Model file for the job. Use its own axes, mm. Face numbers are marked on the shaded views. A direction names the side the tool comes from. Round coordinates to 2 decimals unless told otherwise and drop trailing zeros. Loops run counter-clockwise (first coordinate to the right, second up) from the corner with the lowest first, then second, coordinate; pieces in that order, holes last. Notation, with made-up numbers: (-23.75, -28.75) -> (26.25, -28.75) arc R34 cw to (26.25, 3.25) -> close; hole circle Ø9 at (20, 25). An arc over 180 degrees is marked (long way). Use a Markdown table: item, result. Add a question column.
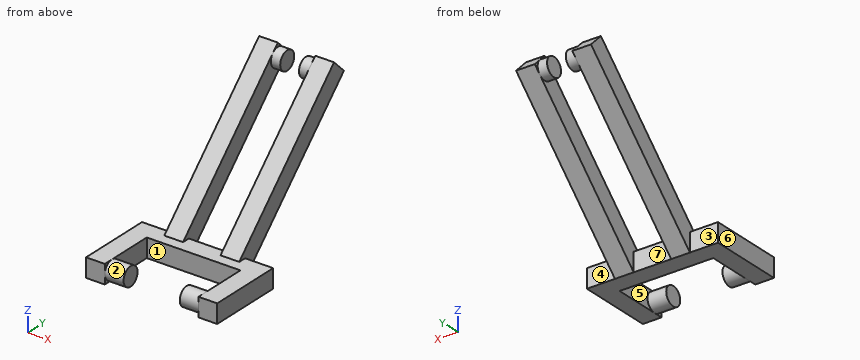
```python
from build123d import *

# Parameters (mm, degrees)
F1_DEPTH = 10
F2_R     = 5
F3_DEPTH = 10
F7_DEPTH = 10
F8_R     = 5
F9_DEPTH = 5


with BuildPart() as f1:
    # F0 (on Top) → F1 (new body)
    with BuildSketch(Plane.XY):
        Polygon((-35, -18.6133389152), (-25, -18.6133389152), (-25, -8.6133389152), (-25, 11.3866610848), (25, 11.3866610848), (25, -8.6133389152), (25, -18.6133389152), (35, -18.6133389152), (35, 21.3866610848), (-35, 21.3866610848), align=None)
    extrude(amount=F1_DEPTH)

    # F2 (on face) → F3 (join)
    with BuildSketch(Plane.YZ.offset(-25)):
        with Locations((-13.5789485648, 5)):
            Circle(F2_R)
    extrude(amount=F3_DEPTH)

    # F4: F1 across plane


with BuildPart() as f1_1:
    add(f1.part)
    add(f1.part.mirror(Plane.YZ))

    # F6 (on offset) → F7 (join)
    with BuildSketch(Plane.YZ.offset(10)):
        Polygon((14.3155932729, 7.0710678119), (21.3866610848, 0), (92.0973392034, 70.7106781187), (85.0262713916, 77.7817459305), align=None)
    extrude(amount=F7_DEPTH)

    # F8 (on face) → F9 (join)
    with BuildSketch(Plane(origin=(10, 0, 0), x_dir=(0, -1, 0), z_dir=(-1, 0, 0))):
        with Locations((-85.0262713916, 70.7106781187)):
            Circle(F8_R)
    extrude(amount=F9_DEPTH)

    # F10: F1 across plane


with BuildPart() as f1_2:
    add(f1_1.part)
    add(f1_1.part.mirror(Plane.YZ))


solid = f1_2.part
```
1) Cut at A-A on x = -17.5. Write the cut outline in (y, z).
2) Cut at C-C on z = 22. Write the cut outline in (x, y), and give its area (3 significant figures).
3) Pull direction Y, two halves, no side cores. Call the marked faces 5, 6 and 7: +Y half, -Y half, draft (parallel to the pull), parting line (faces both ways), or undercut.
4) Cut at B-B on y = -4.5. Write the cut outline in (x, z).
5) Wall check: probe 1 along X at (y, z) = (29.5, 17.5); probe 2 along X at (y, z) = (5.5, 5); probe 3 along Z at (x, y) = (28, 18.5). Give the ranges that are in metal, low to high. Write a range as from..to.
6) Pin check, flat tips, straight feed: pin 1 Ø2 at (x, z) = (-21.5, 66.5) entering from -Y; pin 2 Ø5 at (x, z) = (-7.5, 7) entering from -Y; pin 3 Ø8 at (x, z) = (-2.5, 4.5) entering from +Y; pin 4 Ø12 at (x, y) = (11, 46) entering from -Z. Stop position of each tip, or through.
7) Tool access for the marked faces 1, 2, 3 and 4: list every direction of +Z, -Z, +X, -X, +Y, -Y with a clear straight run to the whole face (end or side of a thin tool).
Established:
| question | item | result |
|---|---|---|
| 1 | outline | circle Ø10 at (-13.58, 5); (11.39, 0) -> (21.39, 0) -> (92.1, 70.71) -> (85.03, 77.78) -> (17.24, 10) -> (11.39, 10) -> close |
| 2 | outline | (-20, 29.24) -> (-10, 29.24) -> (-10, 43.39) -> (-20, 43.39) -> close; (10, 29.24) -> (20, 29.24) -> (20, 43.39) -> (10, 43.39) -> close |
| 2 | area | 283 mm^2 |
| 3 | face 5 | undercut |
| 3 | face 6 | draft |
| 3 | face 7 | +Y half |
| 4 | outline | (-35, 0) -> (-25, 0) -> (-25, 10) -> (-35, 10) -> close; (25, 0) -> (35, 0) -> (35, 10) -> (25, 10) -> close |
| 5 | probe 1 | x = -20..-10, 10..20 |
| 5 | probe 2 | x = -35..-25, 25..35 |
| 5 | probe 3 | z = 0..10 |
| 6 | pin 1 | passes through |
| 6 | pin 2 | stops at y = 11.39 |
| 6 | pin 3 | stops at y = 21.39 |
| 6 | pin 4 | stops at z = 18.61 |
| 7 | face 1 | +Z, -Z |
| 7 | face 2 | none |
| 7 | face 3 | +Z, -Z, -X, +Y |
| 7 | face 4 | +Z, -Z, +X, +Y |
